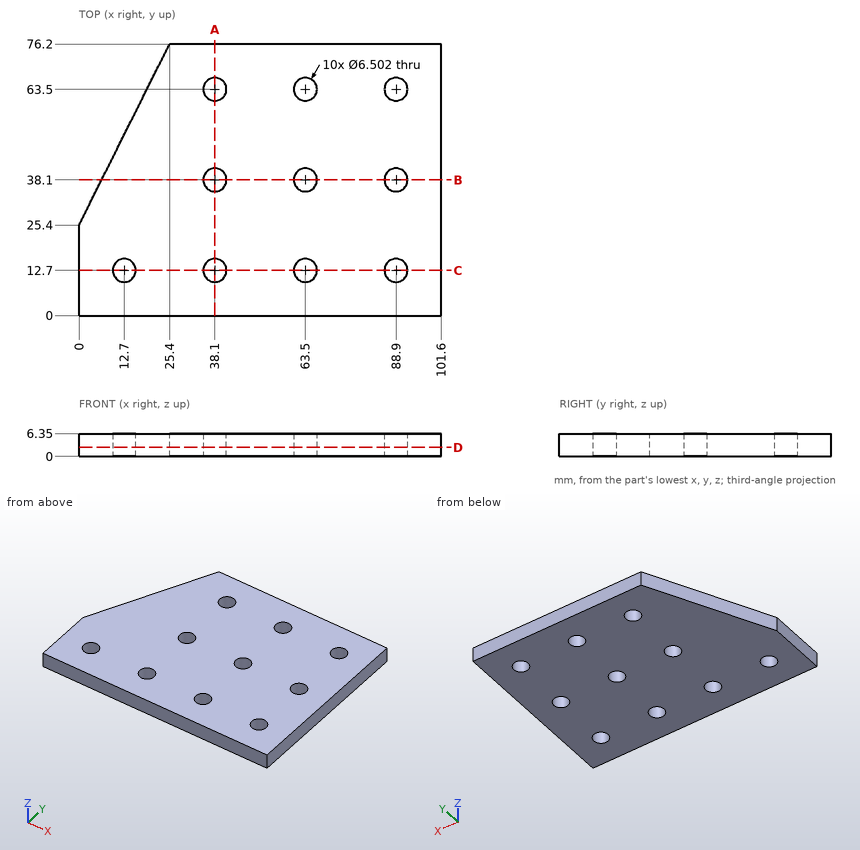
Answer from the drawing. Dimensions are ordinates in mm from the lowest x, y and z of the part. Round coordinates to 2 decimals unless told otherwise and drop trailing zeros. Write each loop counter-clockwise with the first axis right and the second up, starting at its lowest first coordinate (ties: lowest second). Pieces come first, ordered by that corner, then holes. Notation, with made-up numbers: M 60,83.5 L 68,83.5 A27 cw 68,107.5 Z; hole C 67.25,-27 d6. An arc over 180 degrees is marked long. Write each question's results on one line, items separated by ' | '. Start each with the question number.
Item 1: Find section D-D on z = 2.5. Give the number of separate pieces and of enclosed holes in the cut face.
Item 2: Find section B-B on y = 38.1. Write down the section's boundary in (x, z), and give its area (3 significant figures).
Item 3: Find section A-A on x = 38.1. Write down the section's boundary in (y, z), and give its area (3 significant figures).
Item 4: Straight lines are drawn through the part: probe 1 along Y at (x, z) = (38.1, 3); probe 2 along Y at (x, z) = (41, 4); probe 3 along Y at (x, z) = (14.5, 5) (1 decimal). For each, find the intervals that lie inside material, in ascending order.
Item 5: Given pin 1 Ø10.5 at (x, y) = (38.1, 12.7) entering from +Z, flat-ended and moving along its own axis, determine where the tip first touches the part or whether it passes through.
Item 6: Find section C-C on y = 12.7. Write down the section's boundary in (x, z), and give its area (3 significant figures).
Answer block:
1) separate pieces: 1 | enclosed holes: 10
2) outline: M 6.35,0 L 34.85,0 L 34.85,6.35 L 6.35,6.35 Z; M 41.35,0 L 60.25,0 L 60.25,6.35 L 41.35,6.35 Z; M 66.75,0 L 85.65,0 L 85.65,6.35 L 66.75,6.35 Z; M 92.15,0 L 101.6,0 L 101.6,6.35 L 92.15,6.35 Z | area: 481 mm²
3) outline: M 0,0 L 9.45,0 L 9.45,6.35 L 0,6.35 Z; M 15.95,0 L 34.85,0 L 34.85,6.35 L 15.95,6.35 Z; M 41.35,0 L 60.25,0 L 60.25,6.35 L 41.35,6.35 Z; M 66.75,0 L 76.2,0 L 76.2,6.35 L 66.75,6.35 Z | area: 360 mm²
4) probe 1: y = 0 to 9.45, 15.95 to 34.85, 41.35 to 60.25, 66.75 to 76.2 | probe 2: y = 0 to 11.23, 14.17 to 36.63, 39.57 to 62.03, 64.97 to 76.2 | probe 3: y = 0 to 10, 15.4 to 54.4
5) pin 1: stops at z = 6.35
6) outline: M 0,0 L 9.45,0 L 9.45,6.35 L 0,6.35 Z; M 15.95,0 L 34.85,0 L 34.85,6.35 L 15.95,6.35 Z; M 41.35,0 L 60.25,0 L 60.25,6.35 L 41.35,6.35 Z; M 66.75,0 L 85.65,0 L 85.65,6.35 L 66.75,6.35 Z; M 92.15,0 L 101.6,0 L 101.6,6.35 L 92.15,6.35 Z | area: 480 mm²
